Source: CAD feature listing. Evaluate the final solid. Frame: model axes, mm. Face numbers are marked on the shaded views. Give positions to 0.01 mm unless a question says otherwise; leave off trailing zeros. Order: outer loops, then holes, each group sorted by start corner. A loop starts at its lowest first (then second) coordinate and runs counter-clockwise, first axis right, second up. Notation, with made-up numbers: (82, -27) - (96, -27) arc R10 ccw to (96, -23) - close; hole circle Ø2 at (41.5, 25.5). An arc over 180 degrees is marked (long way). Answer as CSV lines item,"result".
```python
from build123d import *

# Parameters (mm, degrees)
F1_DEPTH    = 3
F2_R        = 5.6
F3_DEPTH    = 2
F5_DEPTH    = 10
F7_DEPTH    = 3
F8_R        = 2.99999
F9_T1_DEPTH = 35
F9_T4_ANGLE = 180
F9_T6_ANGLE = 180


# Not quite as in the source:
# - a fillet or chamfer that OpenCascade refuses, or shapes differently, is made with other operations: its cross-section is extruded or revolved along the edge and cut away or added
# - a fillet or chamfer is up to 0.001 mm smaller than in the source, because OpenCascade refuses the exact size


with BuildPart() as f1:
    # F0 (on Top) → F1 (new body)
    with BuildSketch(Plane.XY):
        with BuildLine():
            Line((14, -17.5), (14, 17.5))
            ThreePointArc((14, 17.5), (0, 31.5), (-14, 17.5))
            Line((-14, 17.5), (-14, -17.5))
            ThreePointArc((-14, -17.5), (0, -31.5), (14, -17.5))
        make_face()
    extrude(amount=F1_DEPTH)

    # F2 (on face) → F3 (cut)
    with BuildSketch(Plane.XY.offset(3)):
        with Locations((0, 17.5)):
            Circle(F2_R)
        with Locations((0, -17.5)):
            Circle(F2_R)
    extrude(amount=-F3_DEPTH, mode=Mode.SUBTRACT)

    # F4 (on Top) → F5 (join)
    with BuildSketch(Plane.XY):
        with BuildLine():
            Line((-11, -26.1602540378), (-11, 26.1602540378))
            ThreePointArc((-11, 26.1602540378), (-13.2287565553, 22.082575695), (-14, 17.5))
            Line((-14, 17.5), (-14, -17.5))
            ThreePointArc((-14, -17.5), (-13.2287565553, -22.082575695), (-11, -26.1602540378))
        make_face()
        Polygon((14, -11.5172988935), (14, 11.5172988935), (11, 9), (11, -9), align=None)
    extrude(amount=F5_DEPTH)

    # F6 (on face) → F7 (join)
    with BuildSketch(Plane.XY.offset(10)):
        with BuildLine():
            Line((14, -17.5), (14, 17.5))
            ThreePointArc((14, 17.5), (4.582575695, 30.7287565553), (-11, 26.1602540378))
            Line((-11, 26.1602540378), (-11, -26.1602540378))
            ThreePointArc((-11, -26.1602540378), (4.582575695, -30.7287565553), (14, -17.5))
        make_face()
        with BuildLine():
            Line((-11, -26.1602540378), (-11, 26.1602540378))
            ThreePointArc((-11, 26.1602540378), (-13.2287565553, 22.082575695), (-14, 17.5))
            Line((-14, 17.5), (-14, -17.5))
            ThreePointArc((-14, -17.5), (-13.2287565553, -22.082575695), (-11, -26.1602540378))
        make_face()
    extrude(amount=F7_DEPTH)

    # F8 (radius 3 in the source; OpenCascade refuses exactly that, so slightly less here)
    f8_edges = [f1.edges().sort_by_distance(p)[0] for p in [
        (14, 0, 13),
        (0, 31.5, 13),
        (-14, 0, 13),
        (0, -31.5, 13),
    ]]
    fillet(f8_edges, radius=F8_R)

    # F9: fillet of radius 5 on 4 edges, made by hand

    # F9_s2 → F9_t1 (cut)
    with BuildSketch(Plane.XZ.offset(-17.5)):
        with BuildLine():
            ThreePointArc((14, 5), (12.5355339059, 1.4644660941), (9, 0))
            Line((9, 0), (14, 0))
            Line((14, 0), (14, 5))
        make_face()
        with BuildLine():
            ThreePointArc((-9, 0), (-12.5355339059, 1.4644660941), (-14, 5))
            Line((-14, 5), (-14, 0))
            Line((-14, 0), (-9, 0))
        make_face()
    extrude(amount=F9_T1_DEPTH, mode=Mode.SUBTRACT)

    # F9_s3 → F9_t4 (revolve, cut)
    with BuildSketch(Plane.XZ.offset(17.5)):
        with BuildLine():
            ThreePointArc((14, 5), (12.5355339059, 1.4644660941), (9, 0))
            Line((9, 0), (14, 0))
            Line((14, 0), (14, 5))
        make_face()
    revolve(axis=Axis((0, -17.5, 0), (0, 0, -1)), revolution_arc=F9_T4_ANGLE, mode=Mode.SUBTRACT)

    # F9_s5 → F9_t6 (revolve, cut)
    with BuildSketch(Plane.XZ.offset(-17.5)):
        with BuildLine():
            ThreePointArc((-14, 5), (-12.5355339059, 1.4644660941), (-9, 0))
            Line((-9, 0), (-14, 0))
            Line((-14, 0), (-14, 5))
        make_face()
    revolve(axis=Axis((0, 17.5, 0), (0, 0, -1)), revolution_arc=F9_T6_ANGLE, mode=Mode.SUBTRACT)


solid = f1.part
```
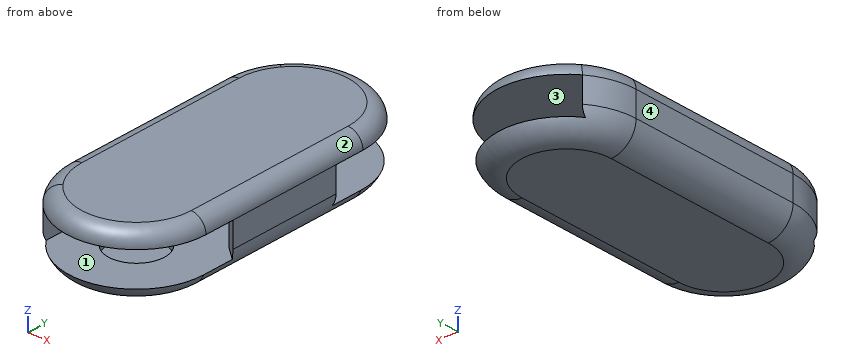
(1) Mould query, pull axis Z, two halves, no side actions, for the marked faces 1, 2, 3 and 4. Classes: released by +Z, released by -Z, zero draft, split by the parting line, or undercut.
Completed:
face 1,"undercut"
face 2,"released by +Z"
face 3,"undercut"
face 4,"zero draft"
(2) Cut plane B-B (y = 4). Return loops of the section in (x, z), then the cut area to 3 significant figures.
Completed:
outline,"(-14, 5) arc R5 ccw to (-9, 0) - (9, 0) arc R5 ccw to (14, 5) - (14, 10) arc R3 ccw to (11, 13) - (-11, 13) arc R3 ccw to (-14, 10) - close; hole (-11, 3) - (11, 3) - (11, 10) - (-11, 10) - close"
area,"195 mm²"
(3) Cut plane A-A (z = 5.75). Return loops of the section in (x, y), then the cut area to 3 significant figures.
Completed:
outline,"(-14, -17.5) arc R14 ccw to (-11, -26.16) - (-11, 26.16) arc R14 ccw to (-14, 17.5) - close; (11, -9) - (14, -11.52) - (14, 11.52) - (11, 9) - close"
area,"202 mm²"
(4) Ray query, line 1 (Z direction, x = 7, y = 3.5); line 2 (Z direction, x = 0.75, y = -12.5); line 3 (Y direction, x = 0, z = 2.4). Return the intervals inside material, ascending. Write a range as from..to.
Completed:
line 1,"0..3, 10..13"
line 2,"0..1, 10..13"
line 3,"-30.77..-23.1, -11.9..11.9, 23.1..30.77"
(5) Contact query for flat-ended pins moving along their axis: pin 1 (3 mm diameter, centred on y = -14, z = 3.5, fed in from +X); pin 2 (5 mm diameter, centred on y = -21.5, z = 5, fed in from +X); pin 3 (5 mm diameter, centred on y = 21, z = 7, fed in from +X). Output: stop coordinate, or through.
Completed:
pin 1,"x = 13.58"
pin 2,"x = 13.35"
pin 3,"x = -11"
